from build123d import *

# Parameters (mm, degrees)
SKETCH1_W           = 25.4
SKETCH1_H           = 25.4
SKETCH1_W_2         = 22.098
SKETCH1_H_2         = 22.098
BOSS_EXTRUDE1_DEPTH = 158.03712
SKETCH7_W           = 25.4
SKETCH7_H           = 25.4
SKETCH7_W_2         = 22.098
SKETCH7_H_2         = 22.098
BOSS_EXTRUDE2_DEPTH = 12.7
CUT_EXTRUDE1_DEPTH  = 36.4
SKETCH9_W           = 25.4
SKETCH9_H           = 25.4
SKETCH9_W_2         = 22.098
SKETCH9_H_2         = 22.098
BOSS_EXTRUDE3_DEPTH = 25.4
CUT_EXTRUDE2_DEPTH  = 36.4


with BuildPart() as part:
    # Sketch1 → Boss-Extrude1 (new body)
    with BuildSketch(Plane.XY):
        Rectangle(SKETCH1_W, SKETCH1_H)
        Rectangle(SKETCH1_W_2, SKETCH1_H_2, mode=Mode.SUBTRACT)
    extrude(amount=BOSS_EXTRUDE1_DEPTH)

    # Sketch7 → Boss-Extrude2 (add)
    with BuildSketch(Plane(origin=(0, 0, 0), x_dir=(-1, 0, 0), z_dir=(0, 0, -1))):
        Rectangle(SKETCH7_W, SKETCH7_H)
        Rectangle(SKETCH7_W_2, SKETCH7_H_2, mode=Mode.SUBTRACT)
    extrude(amount=BOSS_EXTRUDE2_DEPTH)

    # Sketch8 → Cut-Extrude1 (cut, through all)
    with BuildSketch(Plane(origin=(0, 22.7, 0), x_dir=(1, 0, 0), z_dir=(0, 1, 0))):
        Polygon((42.140856973, 36.508313653), (-34.628433436, -30), (-56.571600074, 82.773791124), align=None)
    extrude(amount=-CUT_EXTRUDE1_DEPTH, mode=Mode.SUBTRACT)

    # Sketch9 → Boss-Extrude3 (add)
    with BuildSketch(Plane.XY.offset(158.037119512)):
        Rectangle(SKETCH9_W, SKETCH9_H)
        Rectangle(SKETCH9_W_2, SKETCH9_H_2, mode=Mode.SUBTRACT)
    extrude(amount=BOSS_EXTRUDE3_DEPTH)

    # Sketch11 → Cut-Extrude2 (cut, through all)
    with BuildSketch(Plane(origin=(-388.03129279, 22.7, 553.337933672), x_dir=(-1, 0, 0), z_dir=(0, 1, 0))):
        Polygon((-356.047433406, -423.010988055), (-328.054453058, -334.045248583), (-413.969286498, -372.828656955), align=None)
    extrude(amount=-CUT_EXTRUDE2_DEPTH, mode=Mode.SUBTRACT)


solid = part.part
The listing builds one solid part. Answer for the finished solid, in the listing's coordinates (mm). A direction names the side the tool comes from. Coordinates: 2 decimals unless noted, no trailing zeros. Order: outer loops, then holes, each group sorted by start corner. A loop starts at its lowest first (then second) coordinate and runs counter-clockwise, first axis right, second up. Notation, with made-up numbers: (-12.5, 75.25) -> (-2.5, 75.25) arc R33 cw to (-2.5, 105.25) -> close; hole circle Ø3 at (-19, 78). An arc over 180 degrees is marked (long way). Answer in a Markdown table with one row per item. Add a question column.
Item 1: Find the intervals of material crossed by L1, parallel to X at y = 2.25, z = 84; L2, parallel to X at y = 6.5, z = -1.5, in increasing order. Write a range as from..to.
Item 2: Determine the mould class of faces 3 (the face through (0, -11.049, 78)), 4 (the face through (0, -12.7, 78)), 5 (the face through (0.178, 11.467, 158.191)) for opening direction Y: +Y half, -Y half, draft (parallel to the pull), parting line (faces both ways), or undercut.
Item 3: Find section B-B (z = 73.5). Write down the section's boundary in (x, y), then the cut area to 3 significant figures.
Item 4: Find section C-C (x = -6.5). Write down the section's boundary in (y, z).
Item 5: Which of the six approach directions +Z, -Z, +X, -X, +Y, -Y give full straight-line access (tool end or side, diameter ignored) to faces 1 (the face through (-12.7, 0, 78)), 2 (the face through (-11.049, 0, 78))?
Item 6: Find section D-D (z = 152). Write down the section's boundary in (x, y), then the cut area to 3 significant figures.
Item 7: Find section A-A (y = -3.75). Write down the section's boundary in (x, z).
Result set:
| question | item | result |
|---|---|---|
| 1 | L1 | x = -12.7..-11.05, 11.05..12.7 |
| 1 | L2 | x = 11.05..12.7 |
| 2 | face 3 | undercut |
| 2 | face 4 | -Y half |
| 2 | face 5 | draft |
| 3 | outline | (-12.7, -12.7) -> (12.7, -12.7) -> (12.7, 12.7) -> (-12.7, 12.7) -> close; hole (-11.05, -11.05) -> (11.05, -11.05) -> (11.05, 11.05) -> (-11.05, 11.05) -> close |
| 3 | area | 157 mm² |
| 4 | outline | (-12.7, 5.63) -> (-11.05, 5.63) -> (-11.05, 152.41) -> (-12.7, 152.41) -> close; (11.05, 5.63) -> (12.7, 5.63) -> (12.7, 152.41) -> (11.05, 152.41) -> close |
| 5 | face 1 | +Z, -Z, -X, +Y, -Y |
| 5 | face 2 | +Z, -Z |
| 6 | outline | (-6.97, -12.7) -> (12.7, -12.7) -> (12.7, 12.7) -> (-6.97, 12.7) -> (-6.97, 11.05) -> (11.05, 11.05) -> (11.05, -11.05) -> (-6.97, -11.05) -> close |
| 6 | area | 101 mm² |
| 7 | outline | (-12.7, 11) -> (-11.05, 9.57) -> (-11.05, 148.46) -> (-12.7, 147.03) -> close; (11.05, -9.57) -> (12.7, -11) -> (12.7, 169.04) -> (11.05, 167.61) -> close |
